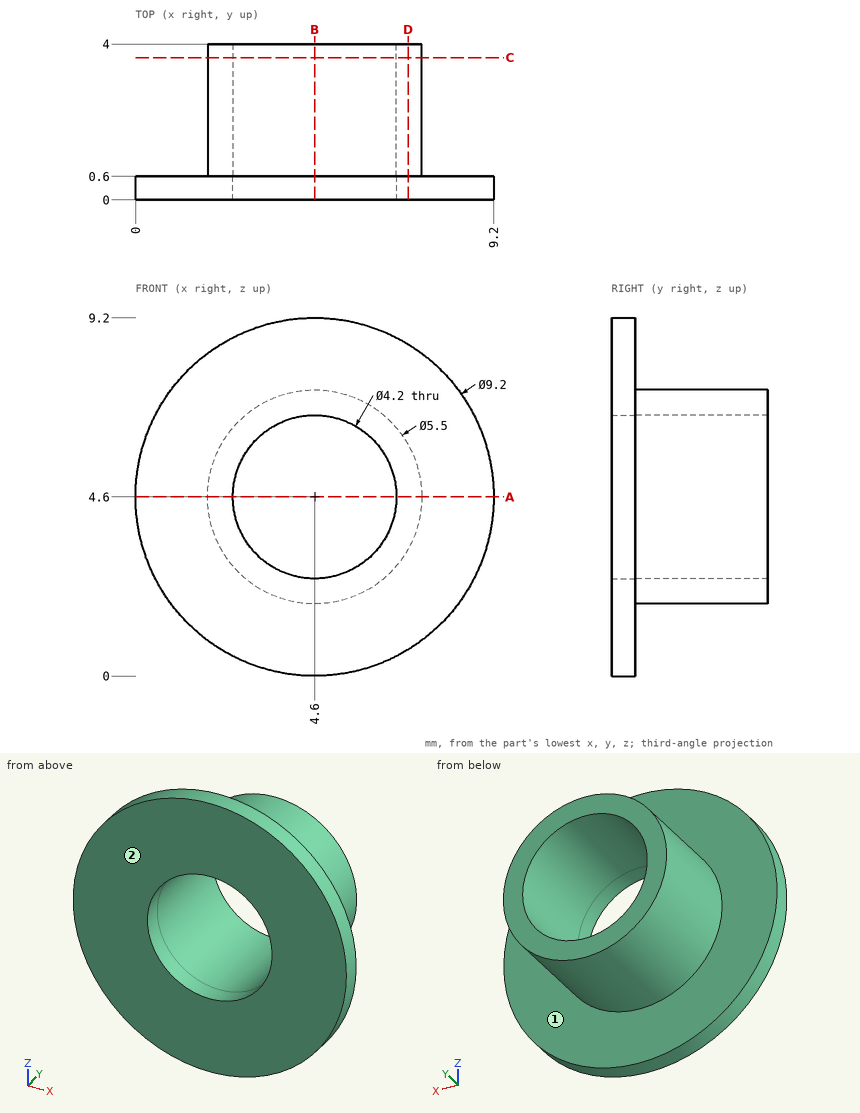
Print and shaded views of the part. All mm, measured from the part's lowest x, y and z. A direction names the side the tool comes from. Give positions to 0.01 mm unless a question says otherwise; leave off trailing zeros. Order: outer loops, then holes, each group sorted by start corner. A loop starts at its lowest first (then second) coordinate and runs counter-clockwise, first axis right, second up. Notation, with made-up numbers: (61, -36) -> (119, -36) arc R6 ccw to (119, -26) -> close; hole circle Ø4 at (80.25, 70.25). An arc over 180 degrees is marked (long way). Use CSV: the item, a comma, the result in double quotes.
1. Drill centre lines: line 1 along Z through (x, y) = (4.6, 1.75); line 2 along X through (y, z) = (0.25, 4.6). Where is each one in solid material? Low to high. Write a range as from..to.
Outcome:
line 1,"1.85..2.5, 6.7..7.35"
line 2,"0..2.5, 6.7..9.2"
2. Band-saw the part on A-A, the plane z = 4.6. Give the cut face in (x, y).
Outcome:
outline,"(0, 0) -> (2.5, 0) -> (2.5, 4) -> (1.85, 4) -> (1.85, 0.6) -> (0, 0.6) -> close; (6.7, 0) -> (9.2, 0) -> (9.2, 0.6) -> (7.35, 0.6) -> (7.35, 4) -> (6.7, 4) -> close"
3. Band-saw the part on D-D, the plane x = 7. Give the cut face in (y, z).
Outcome:
outline,"(0, 0.68) -> (0.6, 0.68) -> (0.6, 3.26) -> (4, 3.26) -> (4, 5.94) -> (0.6, 5.94) -> (0.6, 8.52) -> (0, 8.52) -> close"
4. Band-saw the part on C-C, the plane y = 3.65. Give the cut face in (x, z), then the cut area to 3 significant figures.
Outcome:
outline,"circle Ø5.5 at (4.6, 4.6); hole circle Ø4.2 at (4.6, 4.6)"
area,"9.90 mm²"
5. Band-saw the part on B-B, the plane x = 4.6. Give the cut face in (y, z).
Outcome:
outline,"(0, 0) -> (0.6, 0) -> (0.6, 1.85) -> (4, 1.85) -> (4, 2.5) -> (0, 2.5) -> close; (0, 6.7) -> (4, 6.7) -> (4, 7.35) -> (0.6, 7.35) -> (0.6, 9.2) -> (0, 9.2) -> close"
6. 3-axis set-ups, long thin cutter, end or side, ignore diameter. For the marked faces 1 and 2: which of +Z, -Z, +X, -X, +Y, -Y reach the whole face in a straight line?
Outcome:
face 1,"+Y"
face 2,"+Z, -Z, +X, -X, -Y"
7. Drop a flat-ended pin along its axis: pin 1 (1.5 mm diameter, centred on x = 3, y = 1, fed in from +Z). Give the stop position or say it passes through.
Outcome:
pin 1,"z = 9.1"
